Could you check a few things on this model? Use its own coordinates, in mm. Face numbers are marked on the shaded views. A direction names the side the tool comes from. Round coordinates to 2 decimals unless told otherwise and drop trailing zeros. Write each loop counter-clockwise with the first axis right and the second up, starting at its lowest first coordinate (ties: lowest second). Pieces come first, ordered by that corner, then holes. Notation, with made-up numbers: (-20.5, -3.5) - (-12.5, -3.5) arc R31 ccw to (-12.5, 28.5) - close; hole circle Ø1 at (28.25, 38.5). An arc over 180 degrees is marked (long way). Write each question's results on one line, items separated by ' | '. Start each with the question number.
(1) For P1, Ø8, axis at x = -439.5, y = 7, coming from the +Z side; P2, Ø5, axis at x = -290.5, y = 5, coming from the +Z side; P3, Ø5, axis at x = -325.5, z = 8, coming from the +Y side, each with a flat end and sliding along its axis, tell me the tip position at first contact or that it passes through.
(2) Imagine slicing it at C-C on z = 9. Write out the boundary of the cut face in (x, y), then the cut area to 3 significant figures.
(3) Please list where these lines run through material, in increasing order: line 1 (Y direction, x = -419, z = 4.75); line 2 (X direction, y = 14.5, z = 1). Write a range as [from, to].
(4) Imagine slicing it at B-B on y = 31.5. Write out the boundary of the cut face in (x, z).
(5) Imagine slicing it at A-A on x = -348. Write out the boundary of the cut face in (y, z), then the cut area to 3 significant figures.
(6) On a 3-axis mill with a long thin cutter (end or side, diameter ignored), from which of +Z, -Z, +X, -X, +Y, -Y can I reach the whole of each face in a straight line? I mean the marked faces 1 and 2. Say none if no direction works.
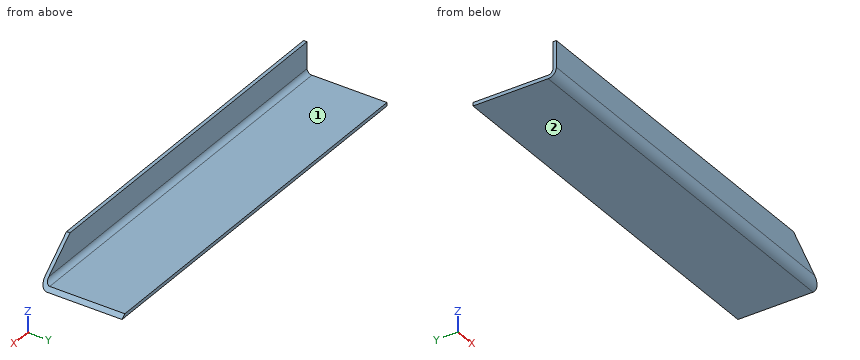
Autodesk Inventor part; units mm, degrees
ref_plane "YZ Plane" through (0, 0, 0) normal (1, 0, 0) x (0, 1, 0)
ref_plane "XZ Plane" through (0, 0, 0) normal (0, 1, 0) x (-1, 0, 0)
ref_plane "XY Plane" through (0, 0, 0) normal (0, 0, 1) x (1, 0, 0)
sketch "Sketch1" plane through (0, 0, 0) normal (0, 0, 1) x (1, 0, 0)
  line L0 (-490, 48) -> (490, 48)
  line L1 (490, 48) -> (490, 0)
  line L2 (490, 0) -> (-490, 0)
  line L3 (-490, 0) -> (-490, 48)
  point P0 (0, 0)
  point P1 (0, 0)
  dimension "d0" = 980
  dimension "d1" = 48
extrude "Plate1" add sketch "Sketch1" along normal blind 2
sketch "Sketch2" plane through (490, 2, 0) normal (0, -1, 0) x (1, 0, 0)
  line L0 (-980, 0) -> (0, 0)
  line L1 (0, 0) -> (0, 20)
  line L2 (0, 20) -> (-980, 20)
  line L3 (-980, 20) -> (-980, 0)
edge flange "Flange1" height 20 angle 90 thickness 2 bend radius 2.75 thickness toward (0, -1, 0) relief round relief width 2 relief depth 1 edges at (0, 0, 2) wall of the first edge with corners at (-490, 2, 0) (490, 2, 0) (490, 2, 20) (-490, 2, 20)
bend "Bend1"
corner "Corner1"
sketch "Sketch5" plane through (0, 0, 0) normal (0, 0, -1) x (-1, 0, 0)
  line L0 (490, 48) -> (-490, 48)
  line L1 (490, 0) -> (-490, 0)
  circle A0 centre (0, 48) radius 35
  line L2 (243.95, 48) -> (246.05, 48)
  line L3 (246.05, 48) -> (246.05, 27)
  line L4 (246.05, 27) -> (243.95, 27)
  line L5 (243.95, 27) -> (243.95, 48)
  line L6 (-243.95, 48) -> (-246.05, 48)
  line L7 (-246.05, 48) -> (-246.05, 27)
  line L8 (-246.05, 27) -> (-243.95, 27)
  line L9 (-243.95, 27) -> (-243.95, 48)
  line L10 (0, 48) -> (0, 0) construction
  line L11 (490, 0) -> (490, 48)
  line L12 (-490, 0) -> (-490, 48)
  circle A1 centre (-490, 48) radius 35
  circle A2 centre (490, 48) radius 35
  point P0 (0, 0)
  point P1 (245, 27)
  point P2 (-245, 27)
  point P3 (246.05, 48)
  point P4 (-35, 48)
  point P5 (35, 48)
  point P6 (-246.05, 48)
  point P7 (455, 48)
  point P8 (490, 13)
  point P9 (-490, 13)
  point P10 (-455, 48)
  dimension "d45" = 70
  dimension "d48" = 2.1
  dimension "d49" = 490
  dimension "d51" = 27
  dimension "d52" = 21
extrude "Extrusion1" cut sketch "Sketch5" against normal through all contours L3 L4 L5 L0 | L9 L8 L7 L0
sketch "Sketch9" plane through (0, 0, 2) normal (0, 0, 1) x (1, 0, 0)
  line L0 (-266.5915, 24.3045) -> (-266.5915, 12.3045) construction
  line L1 (-266.5915, 12.3045) -> (-466.5915, 12.3045) construction
  line L2 (-466.5915, 12.3045) -> (-466.5915, 24.3045) construction
  line L3 (-466.5915, 24.3045) -> (-266.5915, 24.3045) construction
  line L4 (-490, 48) -> (490, 48)
  point P0 (0, 0)
  point P1 (1.05, 68)
  point P2 (490, 48)
  dimension "d40" = 200
  dimension "d41" = 12
mark "Mark2"
sketch "Sketch10" plane through (-490, 0, 20) normal (0, -1, 0) x (1, 0, 0)
  line L0 (980, -20) -> (0, -20)
  line L1 (0, 0) -> (980, 0)
  line L2 (980, -20) -> (203.1655, -20)
  line L3 (203.1655, -20) -> (203.1655, 0)
  line L4 (203.1655, 0) -> (980, 0)
  line L5 (980, 0) -> (980, -20)
  line L6 (203.1655, 0) -> (227.0006, -20)
  point P0 (490, -20)
  dimension "d53" = 776.8345
  dimension "d54" = 50
extrude "Extrusion4" cut sketch "Sketch10" along normal through all both and the other way through all contours L0 L6 L1 L5
equation "\"d2\" = Thickness"
equation "\"d3\" = BendReliefWidth"
equation "\"d4\" = BendReliefDepth"
equation "\"d5\" = MinimumRemnant"
equation "\"d6\" = TransitionRadius"
equation "\"d9\" = BendRadius"
equation "\"d10\" = CornerReliefSize"
equation "\"d11\" = GapSize"
equation "\"d12\" = JacobiRadiusSize"
equation "\"BendReliefWidth\" = Thickness"
equation "\"BendReliefDepth\" = 0.5 * Thickness"
equation "\"CornerReliefSize\" = 4 * Thickness"
equation "\"MinimumRemnant\" = 2 * Thickness"
equation "\"TransitionRadius\" = BendRadius"
equation "\"JacobiRadiusSize\" = BendRadius"
equation "\"GapSize\" = Thickness"
properties part number "MSC 327 STRINGER BOARD  ##" material "Stainless Steel"
Response:
1) P1: z = 2.63 | P2: z = 3.17 | P3: y = 2
2) outline: (-490, 0) - (-273.73, 0) - (-273.73, 2) - (-490, 2) - close | area: 433 mm²
3) line 1: [0, 2] | line 2: [-490, -264.19]
4) outline: (-490, 0) - (-263, 0) - (-265.38, 2) - (-490, 2) - close
5) outline: (0, 4.75) arc R4.75 ccw to (4.75, 0) - (48, 0) - (48, 2) - (4.75, 2) arc R2.75 cw to (2, 4.75) - (2, 20) - (0, 20) - close | area: 129 mm²
6) face 1: +Z, +X, -X, +Y | face 2: -Z, +X, -X, +Y, -Y
